```python
from build123d import *

# Parameters (mm, degrees)
SKETCH1_W               = 47
SKETCH1_H               = 30
BOSS_EXTRUDE1_DEPTH     = 14.8
SKETCH2_R               = 5.75
CUT_EXTRUDE1_DEPTH      = 32.564061843
SKETCH10_W              = 15
SKETCH10_H              = 23
BOSS_EXTRUDE2_DEPTH     = 10
SKETCH9_R               = 2.5
CUT_EXTRUDE2_DEPTH      = 52.780787943
SKETCH9_3_W             = 8.89
SKETCH9_3_H             = 8.382
SKETCH9_3_R             = 2.5
CUT_EXTRUDE3_DEPTH      = 28.04
SKETCH14_W              = 11.152996248
SKETCH14_H              = 9.480152006
BOSS_EXTRUDE3_DEPTH     = 11.96
CUT_EXTRUDE6_DEPTH      = 31
CUT_EXTRUDE6_DEPTH_BACK = 111
SKETCH15_R              = 2.5
CHAMFER1_SIZE           = 10
CUT_EXTRUDE7_DEPTH      = 58.99137867
SKETCH17_W              = 15
SKETCH17_H              = 23
CUT_EXTRUDE8_DEPTH      = 10
CUT_EXTRUDE9_DEPTH      = 31.734725749
CUT_EXTRUDE9_DEPTH_BACK = 31.734725749
SKETCH18_R              = 5.75
CUT_EXTRUDE10_START     = -7.3
SKETCH19_R              = 5.75
CUT_EXTRUDE10_DEPTH     = 25.264061843
SKETCH20_W              = 37
SKETCH20_H              = 14.8
SKETCH20_R              = 2.5
BOSS_EXTRUDE4_DEPTH     = 1
BOSS_EXTRUDE5_START     = 1
SKETCH21_W              = 37
SKETCH21_H              = 14.8
SKETCH21_R              = 2.5
BOSS_EXTRUDE5_DEPTH     = 1
BOSS_EXTRUDE6_DEPTH     = 25
CUT_EXTRUDE11_REACH     = 59.065
SKETCH22_W              = 5.115877125
SKETCH22_H              = 1.9
SKETCH24_R              = 2.5
CUT_EXTRUDE12_DEPTH     = 60.960737154
CUT_EXTRUDE13_START     = -19.04
SKETCH25_W              = 9.4
SKETCH25_H              = 8.9
CUT_EXTRUDE13_DEPTH     = 6.08
SKETCH26_W              = 23.327842288
SKETCH26_H              = 8.382
BOSS_EXTRUDE7_DEPTH     = 32
SKETCH27_R              = 3.5
CUT_EXTRUDE14_DEPTH     = 10
SKETCH28_R              = 0.5
BOSS_EXTRUDE8_DEPTH     = 0.5
SKETCH29_W              = 28
SKETCH29_H              = 24
SKETCH29_W_2            = 19.5
SKETCH29_H_2            = 14.8
BOSS_EXTRUDE9_DEPTH     = 53
SKETCH30_W              = 6.5
SKETCH30_H              = 24
BOSS_EXTRUDE10_DEPTH    = 5


with BuildPart() as part:
    # Sketch1 → Boss-Extrude1 (new body)
    with BuildSketch(Plane(origin=(0, 0, 0), x_dir=(1, 0, 0), z_dir=(0, 1, 0))):
        Rectangle(SKETCH1_W, SKETCH1_H)
    extrude(amount=BOSS_EXTRUDE1_DEPTH)

    # Sketch2 → Cut-Extrude1 (cut, through all)
    with BuildSketch(Plane.XZ):
        with Locations(Location((13.5, 0, 0), (0, 0, 270))):
            Circle(SKETCH2_R)
    extrude(amount=-CUT_EXTRUDE1_DEPTH, mode=Mode.SUBTRACT)

    # Sketch10 → Boss-Extrude2 (add)
    with BuildSketch(Plane.XY.offset(15)):
        with Locations((-16, 11.5)):
            Rectangle(SKETCH10_W, SKETCH10_H)
    extrude(amount=BOSS_EXTRUDE2_DEPTH)

    # Sketch9 → Cut-Extrude2 (cut, through all)
    with BuildSketch(Plane.XY.offset(25)):
        with Locations((-16, 4.191)):
            Circle(SKETCH9_R)
    extrude(amount=-CUT_EXTRUDE2_DEPTH, mode=Mode.SUBTRACT)

    # Sketch9<3> → Cut-Extrude3 (cut)
    with BuildSketch(Plane.XY.offset(25)):
        with Locations((-16, 4.191)):
            Rectangle(SKETCH9_3_W, SKETCH9_3_H)
        with Locations((-16, 4.191)):
            Circle(SKETCH9_3_R, mode=Mode.SUBTRACT)
    extrude(amount=-CUT_EXTRUDE3_DEPTH, mode=Mode.SUBTRACT)

    # Sketch14 → Boss-Extrude3 (add)
    with BuildSketch(Plane.XY.offset(15)):
        with Locations((-17.328151157, 4.740076003)):
            Rectangle(SKETCH14_W, SKETCH14_H)
    extrude(amount=-BOSS_EXTRUDE3_DEPTH)

    # Sketch15 → Cut-Extrude6 (cut, two sides: drawn at the far end of the back side and taken through both)
    with BuildSketch(Plane(origin=(0, 0, -15), x_dir=(-1, 0, 0), z_dir=(0, 0, -1)).offset(-CUT_EXTRUDE6_DEPTH_BACK)):
        with Locations(Location((16, 4.191, 0), (0, 0, 180))):
            Circle(SKETCH15_R)
    extrude(amount=CUT_EXTRUDE6_DEPTH + CUT_EXTRUDE6_DEPTH_BACK, mode=Mode.SUBTRACT)

    # Chamfer1
    chamfer1_edges = [part.edges().sort_by_distance(p)[0] for p in [
        (23.5, 7.4, 15),
        (23.5, 7.4, -15),
    ]]
    chamfer(chamfer1_edges, length=CHAMFER1_SIZE)

    # Sketch16 → Cut-Extrude7 (cut, through all)
    with BuildSketch(Plane.ZY.offset(23.5)):
        Polygon((10.175, 14.8), (10.175, 12.9), (14.174668145, 12.951524082), (14.174999863, 11.101524112), (5.675, 11.1), (5.675, 14.8), align=None)
        Polygon((-14.174999863, 11.101524112), (-5.675, 11.1), (-5.675, 14.8), (-10.175, 14.8), (-10.175, 12.9), (-14.174668145, 12.951524082), align=None)
    extrude(amount=-CUT_EXTRUDE7_DEPTH, mode=Mode.SUBTRACT)

    # Sketch17 → Cut-Extrude8 (cut)
    with BuildSketch(Plane.XY.offset(25)):
        with Locations((-16, 11.5)):
            Rectangle(SKETCH17_W, SKETCH17_H)
    extrude(amount=-CUT_EXTRUDE8_DEPTH, mode=Mode.SUBTRACT)

    # Sketch18 → Cut-Extrude9 (cut, two sides: drawn at the far end of the back side and taken through both)
    with BuildSketch(Plane(origin=(2.125798494, 7.933587988, 0), x_dir=(0, 0, 1), z_dir=(0.25881904510252474, 0.9659258262890673, 0)).offset(-CUT_EXTRUDE9_DEPTH_BACK)):
        with Locations((0, 12.699256918)):
            Circle(SKETCH18_R)
    extrude(amount=CUT_EXTRUDE9_DEPTH + CUT_EXTRUDE9_DEPTH_BACK, mode=Mode.SUBTRACT)

    # Sketch19 → Cut-Extrude10 (cut, through all)
    with BuildSketch(Plane(origin=(0, 14.8, 0), x_dir=(1, 0, 0), z_dir=(0, 1, 0)).offset(CUT_EXTRUDE10_START)):
        with Locations((7.08, 0)):
            Circle(SKETCH19_R)
    extrude(amount=-CUT_EXTRUDE10_DEPTH, mode=Mode.SUBTRACT)

    # Sketch20 → Boss-Extrude4 (add)
    with BuildSketch(Plane.XY.offset(15)):
        with Locations((-5, 7.4)):
            Rectangle(SKETCH20_W, SKETCH20_H)
        with Locations((-16, 4.191)):
            Circle(SKETCH20_R, mode=Mode.SUBTRACT)
    extrude(amount=BOSS_EXTRUDE4_DEPTH)

    # Sketch21 → Boss-Extrude5 (add)
    with BuildSketch(Plane(origin=(0, 0, -15), x_dir=(-1, 0, 0), z_dir=(0, 0, -1)).offset(BOSS_EXTRUDE5_START)):
        with Locations((5, 7.4)):
            Rectangle(SKETCH21_W, SKETCH21_H)
        with Locations(Location((16, 4.191, 0), (0, 0, 180))):
            Circle(SKETCH21_R, mode=Mode.SUBTRACT)
    extrude(amount=-BOSS_EXTRUDE5_DEPTH)

    # Sketch23 → Boss-Extrude6 (add)
    with BuildSketch(Plane.ZY.offset(23.5)):
        Polygon((-10.175, 14.8), (-16, 14.8), (-16, 0), (16, 0), (16, 14.8), (10.175, 14.8), (10.175, 12.9), (14.174668145, 12.951524082), (14.174999863, 11.101524112), (5.675, 11.1), (5.675, 14.8), (-5.675, 14.8), (-5.675, 11.1), (-14.174999863, 11.101524112), (-14.174668145, 12.951524082), (-10.175, 12.9), align=None)
    extrude(amount=BOSS_EXTRUDE6_DEPTH)

    # Cut-Extrude11: up to this face of the body (flat: up to its plane)
    cut_extrude11_end = Plane(part.part.faces().sort_by_distance((-2.5875, 13.85, -10.175))[0])
    # Sketch22 → Cut-Extrude11 (cut, up to the picked face)
    with BuildSketch(Plane(origin=(0, 0, 10.175), x_dir=(-1, 0, 0), z_dir=(0, 0, -1)), mode=Mode.PRIVATE) as cut_extrude11_sk1:
        with Locations((-16.601488732, 13.85)):
            Rectangle(SKETCH22_W, SKETCH22_H)
    cut_extrude11_tool1 = split(extrude(cut_extrude11_sk1.sketch, amount=CUT_EXTRUDE11_REACH, mode=Mode.PRIVATE), bisect_by=cut_extrude11_end, keep=Keep.BOTH, mode=Mode.PRIVATE)
    add(cut_extrude11_tool1.solids().sort_by(Axis((16.601489, 13.85, 10.175), (0, 0, -1)))[0], mode=Mode.SUBTRACT)

    # Sketch24 → Cut-Extrude12 (cut, through all)
    with BuildSketch(Plane.XY.offset(16)):
        with Locations((-41, 4.191)):
            Circle(SKETCH24_R)
    extrude(amount=-CUT_EXTRUDE12_DEPTH, mode=Mode.SUBTRACT)

    # Sketch25 → Cut-Extrude13 (cut)
    with BuildSketch(Plane.XY.offset(16).offset(CUT_EXTRUDE13_START)):
        with Locations((-41, 4.191)):
            Rectangle(SKETCH25_W, SKETCH25_H)
    extrude(amount=CUT_EXTRUDE13_DEPTH, mode=Mode.SUBTRACT)

    # Sketch26 → Boss-Extrude7 (add, through all)
    with BuildSketch(Plane.XY.offset(16)):
        with Locations((-16, 4.191)):
            Rectangle(SKETCH26_W, SKETCH26_H)
    extrude(amount=-BOSS_EXTRUDE7_DEPTH)

    # Sketch27 → Cut-Extrude14 (cut)
    with BuildSketch(Plane.XZ.offset(-7.5)):
        with Locations((7.08, 0)):
            Circle(SKETCH27_R)
    extrude(amount=-CUT_EXTRUDE14_DEPTH, mode=Mode.SUBTRACT)

    # Sketch28 → Boss-Extrude8 (add)
    with BuildSketch(Plane(origin=(0, 14.8, 0), x_dir=(1, 0, 0), z_dir=(0, 1, 0))):
        with Locations(Location((-47, 0.175, 0), (0, 0, 90))):
            Circle(SKETCH28_R)
        with Locations(Location((-47, 2.175, 0), (0, 0, 90))):
            Circle(SKETCH28_R)
        with Locations(Location((-47, 4.175, 0), (0, 0, 90))):
            Circle(SKETCH28_R)
    extrude(amount=BOSS_EXTRUDE8_DEPTH)

    # Sketch29 → Boss-Extrude9 (add)
    with BuildSketch(Plane.XZ):
        with Locations((-41, 0)):
            Rectangle(SKETCH29_W, SKETCH29_H)
        with Locations((-41, 0)):
            Rectangle(SKETCH29_W_2, SKETCH29_H_2, mode=Mode.SUBTRACT)
    extrude(amount=BOSS_EXTRUDE9_DEPTH)

    # Sketch30 → Boss-Extrude10 (add)
    with BuildSketch(Plane(origin=(0, 0, 0), x_dir=(1, 0, 0), z_dir=(0, 1, 0))):
        with Locations((-51.75, 0)):
            Rectangle(SKETCH30_W, SKETCH30_H)
    extrude(amount=BOSS_EXTRUDE10_DEPTH)


solid = part.part
```
Source: CAD feature listing. Evaluate the final solid. Frame: model axes, mm. A direction names the side the tool comes from. Coordinates: 2 decimals unless noted, no trailing zeros. Loops run counter-clockwise (first coordinate to the right, second up) from the corner with the lowest first, then second, coordinate; pieces in that order, holes last. Notation, with made-up numbers: (18.5, 9) -> (64.5, 9) arc R31 ccw to (64.5, 47) -> close; hole circle Ø10 at (-12.75, 2). An arc over 180 degrees is marked (long way). One line per item, written item: value. Start each with the question number.
Q1. Section query A-A, the plane x = 7.08. Return the cut outline in (y, z) (3 decimals).
Q2. Section query C-C, the plane x = -41. Give the number of separate pieces and of enclosed holes in the cut face, and give its area (3 significant figures).
Q3. Line query: line 1 along Z through (x, y) = (7, 9); line 2 along Z through (x, y) = (7.08, 1.75); line 3 along X through (y, z) = (3, 0). Output: solid intervals per line, ascending.
Q4. Contact query for flat-ended pins moving along their axis: P1, Ø9.5, axis at x = -3, z = -11.5, coming from the +Y side; P2, Ø10, axis at x = -37, y = -31.5, coming from the -Z side; P3, Ø12, axis at x = -41, y = -17.5, coming from the +Z side; P4, Ø6.5, axis at x = 7.08, z = 0, coming from the +Y side. Output: stop coordinate, or through.
Q5. Set-up query: faces 4 (the face through (11.5, 9.46, 5.39)), 5 (the face through (-15, 14, 10.175)), 6 (the face through (-52, 5, 0)), 7 (the face through (1.333, 3.803, -0.174)). Return all of +Z, -Z, +X, -X, +Y, -Y with unobstructed straight access to the full face (end or side cutting, diameter ignored); none if empty.
Q6. Mould query, pull axis Y, two halves, no side actions, for faces 1 (the face through (-18, 14.8, 0)), 2 (the face through (-38.69, 3.23, 9.61)), 3 (the face through (-17, 7, 16)). Classes: pulls with the +Y half, pulls with the -Y half, needs draft (parallel to the pull), parting line crosses it, or undercut.
Q7. Section query B-B, the plane y = -20. Return the cut outline in (x, z), and give its area (3 significant figures).
Results:
1. outline: (0, -16) -> (14.8, -16) -> (14.8, -10.175) -> (12.9, -10.175) -> (12.952, -14.175) -> (11.102, -14.175) -> (11.1, -5.675) -> (14.8, -5.675) -> (14.8, -3.5) -> (7.5, -3.5) -> (7.5, -5.75) -> (0, -5.75) -> close; (0, 5.75) -> (7.5, 5.75) -> (7.5, 3.5) -> (14.8, 3.5) -> (14.8, 5.675) -> (11.1, 5.675) -> (11.102, 14.175) -> (12.952, 14.175) -> (12.9, 10.175) -> (14.8, 10.175) -> (14.8, 16) -> (0, 16) -> close
2. separate pieces: 3
2. enclosed holes: 0
2. area: 731 mm^2
3. line 1: -16 to -3.5, 3.5 to 16
3. line 2: -16 to -5.75, 5.75 to 16
3. line 3: -55 to -45.7, -36.3 to 1.33, 19.9 to 23.5
4. P1: y = 14.8
4. P2: z = -12
4. P3: z = 12
4. P4: through
5. face 4: +Y, -Y
5. face 5: +X, -X, +Y
5. face 6: +Z, -Z, -X, +Y
5. face 7: -Y
6. face 1: pulls with the +Y half
6. face 2: undercut
6. face 3: needs draft
7. outline: (-55, -12) -> (-27, -12) -> (-27, 12) -> (-55, 12) -> close; hole (-50.75, -7.4) -> (-31.25, -7.4) -> (-31.25, 7.4) -> (-50.75, 7.4) -> close
7. area: 383 mm^2
